```python
from build123d import *

# Parameters (mm, degrees)
SKETCH1_R           = 50
BOSS_EXTRUDE1_DEPTH = 318
SKETCH2_R           = 15
BOSS_EXTRUDE2_DEPTH = 32


with BuildPart() as part:
    # Sketch1 → Boss-Extrude1 (new body)
    with BuildSketch(Plane.XY):
        with Locations((-8.993956806, 14.489721156)):
            Circle(SKETCH1_R)
    extrude(amount=-BOSS_EXTRUDE1_DEPTH)

    # Sketch2 → Boss-Extrude2 (add)
    with BuildSketch(Plane.XY):
        with Locations((-8.993956806, 14.489721156)):
            Circle(SKETCH2_R)
    boss_extrude2 = extrude(amount=BOSS_EXTRUDE2_DEPTH)

    # Mirror1: Boss-Extrude2 across plane
    add(boss_extrude2.mirror(Plane.XY.offset(-159)))


solid = part.part
```
Read the model definition and answer for the solid it produces. Units are mm, in the model's axes. A direction names the side the tool comes from. Coordinates: 2 decimals unless noted, no trailing zeros. Write each loop counter-clockwise with the first axis right and the second up, starting at its lowest first coordinate (ties: lowest second). Pieces come first, ordered by that corner, then holes. Notation, with made-up numbers: (5, 17.25) -> (48, 17.25) arc R24 cw to (48, 55.25) -> close; hole circle Ø5 at (-37.5, -26). An arc over 180 degrees is marked (long way). Answer as a JSON object with one key per item and string values.
Q1. The part is cut by section B-B on x = -17.5. Give the vertices of the cut face in (y, z).
The answers:
{"outline": "(-34.78, -318) -> (2.13, -318) -> (2.13, -350) -> (26.84, -350) -> (26.84, -318) -> (63.76, -318) -> (63.76, 0) -> (26.84, 0) -> (26.84, 32) -> (2.13, 32) -> (2.13, 0) -> (-34.78, 0) -> close"}
Q2. The part is cut by section A-A on y = 23.5. Give the vertices of the cut face in (x, z).
The answers:
{"outline": "(-58.18, -318) -> (-20.99, -318) -> (-20.99, -350) -> (3, -350) -> (3, -318) -> (40.19, -318) -> (40.19, 0) -> (3, 0) -> (3, 32) -> (-20.99, 32) -> (-20.99, 0) -> (-58.18, 0) -> close"}
Q3. The part is cut by section D-D on y = 40.5. Give the vertices of the cut face in (x, z), then the cut area to 3 significant figures.
The answers:
{"outline": "(-51.7, -318) -> (33.71, -318) -> (33.71, 0) -> (-51.7, 0) -> close", "area": "27,200 mm2"}
Q4. The part is cut by section C-C on z = -302.5. Give the vertices of the cut face in (x, y).
The answers:
{"outline": "circle Ø100 at (-8.99, 14.49)"}
Q5. Consider line 1 (Z direction, x = -53, y = -4); line 2 (X direction, y = 55, z = -63.5); line 3 (X direction, y = 6, z = -332). Determine where each line is inside the solid, lowest interval first. Write a range as [from, to].
The answers:
{"line 1": "z = [-318, 0]", "line 2": "x = [-38.3, 20.31]", "line 3": "x = [-21.36, 3.37]"}
Q6. A tool of negligible diameter and unlimited length cuts with its end or side. For faces 1 (the cylindrical face through (-0.93, 27.14, 15.78)), 2 (the cylindrical face through (38.7, 29.5, -156.8)), 3 (the flat face through (-21, 4, -318)), from which of +Z, -Z, +X, -X, +Y, -Y can it reach the whole face along a straight path? Write none if from no direction.
The answers:
{"face 1": "+Z", "face 2": "+Z, -Z", "face 3": "-Z"}
Q7. Flat-ended cylindrical pins translate along their axes: pin 1 Ø3 at (x, y) = (-23.5, 51) entering from +Z; pin 2 Ø5 at (x, z) = (25, -168) entering from +Y; pin 3 Ø3 at (x, y) = (-24.5, 53) entering from -Z. Find the tip coordinate at first contact, or state that the pin passes through.
The answers:
{"pin 1": "stops at z = 0", "pin 2": "stops at y = 53.32", "pin 3": "stops at z = -318"}
